Verification items for the finished model (mm, model axes). Give positions to 0.01 mm unless a question says otherwise; leave off trailing zeros. Order: outer loops, then holes, each group sorted by start corner. A loop starts at its lowest first (then second) coordinate and runs counter-clockwise, first axis right, second up. Notation, with made-up numbers: (15, 30.5) - (68, 30.5) arc R33 cw to (68, 66.5) - close; hole circle Ø1 at (15, -1). An arc over 180 degrees is marked (long way). Answer as a JSON object with one key per item and string values.
```python
from build123d import *

# Parameters (mm, degrees)
EXTRUDE_1_DEPTH     = 10
SKETCH_3_R          = 50
SKETCH_3_R_2        = 40
CUT_EXTRUDE_3_DEPTH = 50


with BuildPart() as part:
    # 草图1 → 凸台-拉伸1 (new body)
    with BuildSketch(Plane.XY):
        with BuildLine():
            Line((-410, 0), (-410, -430))
            Line((-410, -430), (410, -430))
            Line((410, -430), (410, 0))
            ThreePointArc((410, 0), (0, 410), (-410, 0))
        make_face()
    extrude(amount=EXTRUDE_1_DEPTH)

    # 草图3 → 切除-拉伸3 (cut)
    with BuildSketch(Plane.XY.offset(10)):
        with Locations((-130, 270.438352594)):
            Circle(SKETCH_3_R)
        with Locations((130, 270.438352594)):
            Circle(SKETCH_3_R)
        with Locations((-270.562773315, 122.70173436)):
            Circle(SKETCH_3_R_2)
        with Locations((270.562773315, 122.70173436)):
            Circle(SKETCH_3_R_2)
        with BuildLine():
            Line((-130, 0), (-130, -430))
            Line((-130, -430), (130, -430))
            Line((130, -430), (130, 0))
            ThreePointArc((130, 0), (0, 130), (-130, 0))
        make_face()
    extrude(amount=-CUT_EXTRUDE_3_DEPTH, mode=Mode.SUBTRACT)


solid = part.part
```
(1) Section check B-B (z = 3.5). Record the cut outline in (x, y), then the cut area to 3 significant figures.
Computed values:
{"outline": "(-410, -430) - (-130, -430) - (-130, 0) arc R130 cw to (130, 0) - (130, -430) - (410, -430) - (410, 0) arc R410 ccw to (-410, 0) - close; hole circle Ø80 at (-270.56, 122.7); hole circle Ø100 at (-130, 270.44); hole circle Ø100 at (130, 270.44); hole circle Ø80 at (270.56, 122.7)", "area": "453,000 mm²"}
(2) Section check A-A (y = -279). Record the cut outline in (x, z).
Computed values:
{"outline": "(-410, 0) - (-130, 0) - (-130, 10) - (-410, 10) - close; (130, 0) - (410, 0) - (410, 10) - (130, 10) - close"}
(3) Section check C-C (x = 99). Record the cut outline in (y, z).
Computed values:
{"outline": "(84.26, 0) - (231.21, 0) - (231.21, 10) - (84.26, 10) - close; (309.67, 0) - (397.87, 0) - (397.87, 10) - (309.67, 10) - close"}
(4) Gauge pin test, flat end, axial feed: pin 1 Ø2 at (x, z) = (-17.5, 3.5) entering from -Y. Record the tip position at first contact, or that the pin passes through.
Computed values:
{"pin 1": "stops at y = 128.68"}
(5) Section check D-D (x = 0). Record the cut outline in (y, z).
Computed values:
{"outline": "(130, 0) - (410, 0) - (410, 10) - (130, 10) - close"}
(6) Material ranges on line 1 along X through (y, z) = (-363, 4.5); line 2 along X through (y, z) = (63.5, 2); line 3 along Y through (x, z) = (240, 4.75), recorded low to high. Write a range as [from, to].
Computed values:
{"line 1": "x = [-410, -130], [130, 410]", "line 2": "x = [-405.05, -113.44], [113.44, 405.05]", "line 3": "y = [-430, 96.9], [148.51, 332.42]"}
(7) Release check for a two-part mould opening along X. For faces 1 (the cylindrical face through (9, 409.9, 4.9)), 2 (the cylindrical face through (119.161, 221.627, 5.07)), 3 (the flat face through (-97, 89, 0)) record: pulls with the +X half, pulls with the -X half, needs draft (parallel to the pull), parting line crosses it, or undercut.
Computed values:
{"face 1": "parting line crosses it", "face 2": "undercut", "face 3": "needs draft"}
